Here's how the part is built. I have some questions about the finished solid (model axes, mm). Face numbers are marked on the shaded views. A direction names the side the tool comes from. Round coordinates to 2 decimals unless told otherwise and drop trailing zeros. Order: outer loops, then holes, each group sorted by start corner. A loop starts at its lowest first (then second) coordinate and runs counter-clockwise, first axis right, second up. Notation, with made-up numbers: (78.25, 89.25) -> (126.25, 89.25) arc R23 cw to (126.25, 117.25) -> close; hole circle Ø2 at (-38.5, 7). An arc over 180 degrees is marked (long way). One line per item, written item: value.
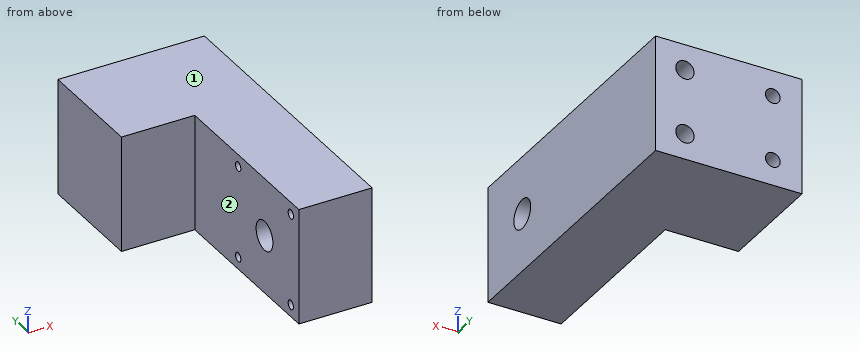
```python
from build123d import *

# Parameters (mm, degrees)
SKETCH1_W                 = 20
SKETCH1_H                 = 31.7
BOSS_EXTRUDE1_DEPTH       = 80
CUT_EXTRUDE1_REACH        = 22
SKETCH2_R                 = 4
M3X0_5_TAPPED_HOLE1_D     = 2.5
M3X0_5_TAPPED_HOLE1_DEPTH = 7.5
M3X0_5_TAPPED_HOLE1_TIP   = 0.751075774
SKETCH5_W                 = 31.7
SKETCH5_H                 = 30.344547228
BOSS_EXTRUDE2_DEPTH       = 20
F_4_0MM_DOWEL_HOLE1_D     = 4
F_4_0MM_DOWEL_HOLE1_DEPTH = 5.2
F_4_0MM_DOWEL_HOLE1_TIP   = 1.201721238
M6X1_0_TAPPED_HOLE1_D     = 5
M6X1_0_TAPPED_HOLE1_DEPTH = 15
M6X1_0_TAPPED_HOLE1_TIP   = 1.502151548


with BuildPart() as part:
    # Sketch1 → Boss-Extrude1 (new body)
    with BuildSketch(Plane(origin=(0, 0, 0), x_dir=(1, 0, 0), z_dir=(0, 1, 0))):
        with Locations((5.656892123, -4.053125)):
            Rectangle(SKETCH1_W, SKETCH1_H)
    extrude(amount=BOSS_EXTRUDE1_DEPTH)

    # Sketch2 → Cut-Extrude1 (cut, up to next)
    with BuildSketch(Plane.ZY.offset(4.343107877), mode=Mode.PRIVATE) as cut_extrude1_sk1:
        with Locations((4.053125, 16.390354737)):
            Circle(SKETCH2_R)
    cut_extrude1_tool1 = extrude(cut_extrude1_sk1.sketch, amount=-CUT_EXTRUDE1_REACH, mode=Mode.PRIVATE) & part.part
    add(cut_extrude1_tool1.solids().sort_by_distance((-4.343108, 16.390355, 4.053125))[0], mode=Mode.SUBTRACT)

    # M3x0.5 Tapped Hole1
    with Locations(Plane.ZY.offset(4.343107877)):
        with Locations((16.604270366, 28.941500103), (-8.498020366, 28.941500103), (-8.498020366, 3.839209371), (16.604270366, 3.839209371)):
            Hole(M3X0_5_TAPPED_HOLE1_D / 2, depth=M3X0_5_TAPPED_HOLE1_DEPTH)
            with Locations((0, 0, -(M3X0_5_TAPPED_HOLE1_DEPTH + M3X0_5_TAPPED_HOLE1_TIP / 2))):  # 118° drill point
                Cone(0, M3X0_5_TAPPED_HOLE1_D / 2, M3X0_5_TAPPED_HOLE1_TIP, mode=Mode.SUBTRACT)

    # Sketch5 → Boss-Extrude2 (add)
    with BuildSketch(Plane.ZY.offset(4.343107877)):
        with Locations((4.053125, 64.827726386)):
            Rectangle(SKETCH5_W, SKETCH5_H)
    extrude(amount=BOSS_EXTRUDE2_DEPTH)

    # Ø4.0mm Dowel Hole1
    with Locations(Plane(origin=(0, 80, 0), x_dir=(1, 0, 0), z_dir=(0, 1, 0))):
        with Locations((-16.343107877, 4.796875), (-16.343107877, -12.903125)):
            Hole(F_4_0MM_DOWEL_HOLE1_D / 2, depth=F_4_0MM_DOWEL_HOLE1_DEPTH)
            with Locations((0, 0, -(F_4_0MM_DOWEL_HOLE1_DEPTH + F_4_0MM_DOWEL_HOLE1_TIP / 2))):  # 118° drill point
                Cone(0, F_4_0MM_DOWEL_HOLE1_D / 2, F_4_0MM_DOWEL_HOLE1_TIP, mode=Mode.SUBTRACT)

    # M6x1.0 Tapped Hole1
    with Locations(Plane(origin=(0, 80, 0), x_dir=(1, 0, 0), z_dir=(0, 1, 0))):
        with Locations((7.656892123, 4.796875), (7.656892123, -12.903125)):
            Hole(M6X1_0_TAPPED_HOLE1_D / 2, depth=M6X1_0_TAPPED_HOLE1_DEPTH)
            with Locations((0, 0, -(M6X1_0_TAPPED_HOLE1_DEPTH + M6X1_0_TAPPED_HOLE1_TIP / 2))):  # 118° drill point
                Cone(0, M6X1_0_TAPPED_HOLE1_D / 2, M6X1_0_TAPPED_HOLE1_TIP, mode=Mode.SUBTRACT)


solid = part.part
```
Q1. I want a section at C-C on x = -13. Write out the boundary of the cut face in (y, z).
Answers:
outline: (49.66, -11.8) -> (80, -11.8) -> (80, 19.9) -> (49.66, 19.9) -> close
Q2. For P1, Ø3, axis at x = -16.34, z = 12.9, coming from the +Y side; P2, Ø5, axis at x = -8, z = -6, coming from the -Y side; P3, Ø3, axis at y = 3.84, z = 16.6, coming from the -X side, each with a flat end and sliding along its axis, tell me the tip position at first contact or that it passes through.
Answers:
P1: y = 74.5
P2: y = 49.66
P3: x = -4.34
Q3. I want a section at A-A on z = 2. Write out the boundary of the cut face in (x, y), then the cut area to 3 significant figures.
Answers:
outline: (-24.34, 49.66) -> (-4.34, 49.66) -> (-4.34, 19.82) -> (15.66, 19.82) -> (15.66, 80) -> (-24.34, 80) -> close; (-4.34, 0) -> (15.66, 0) -> (15.66, 12.96) -> (-4.34, 12.96) -> close
area: 2,070 mm2
Q4. I want a section at B-B on x = 13. Write out the boundary of the cut face in (y, z).
Answers:
outline: (0, -11.8) -> (80, -11.8) -> (80, 19.9) -> (0, 19.9) -> close; hole circle Ø8 at (16.39, 4.05)
Q5. Which directions (+Z, -Z, +X, -X, +Y, -Y) give clear straight access to the entire face, cutting with the end or side of a thin tool? Please do the marked faces 1 and 2.
Answers:
face 1: +Z, +X, -X, +Y, -Y
face 2: +Z, -Z, -X, -Y
Q6. I need wall thicknesses on line 1 along X through (y, z) = (36, -9.5); line 2 along Y through (x, z) = (-19, 1); line 3 along X through (y, z) = (76.5, -6.5). Which ranges of each line are inside material? Lowest first, please.
Answers:
line 1: -4.34 to 15.66
line 2: 49.66 to 80
line 3: -24.34 to -17.39, -15.29 to 5.83, 9.49 to 15.66
Q7. I want a section at D-D on y = 42. Write out the boundary of the cut face in (x, z), then the cut area to 3 significant figures.
Answers:
outline: (-4.34, -11.8) -> (15.66, -11.8) -> (15.66, 19.9) -> (-4.34, 19.9) -> close
area: 634 mm2
